```python
from build123d import *

# Parameters (mm, degrees)
SKETCH005_W     = 13
SKETCH005_H     = 11.2
SKETCH005_W_2   = 11.8
SKETCH005_H_2   = 10
PAD003_DEPTH    = 9.8
FILLET005_R     = 0.3
FILLET006_R     = 0.4
SKETCH006_W     = 1.85
SKETCH006_H     = 0.95
POCKET002_DEPTH = 0.6
FILLET007_R     = 0.13
SKETCH007_R     = 0.3
PAD004_DEPTH    = 1.3


with BuildPart() as part:
    # Sketch005 → Pad003 (new body)
    with BuildSketch(Plane.XY):
        with Locations((0, -1.6)):
            Rectangle(SKETCH005_W, SKETCH005_H)
        with Locations((0, -1.6)):
            Rectangle(SKETCH005_W_2, SKETCH005_H_2, mode=Mode.SUBTRACT)
    extrude(amount=PAD003_DEPTH)

    # Fillet005
    fillet005_edges = [part.edges().sort_by_distance(p)[0] for p in [
        (-6.5, 4, 4.9),
        (-6.5, -7.2, 4.9),
        (6.5, -7.2, 4.9),
        (6.5, 4, 4.9),
    ]]
    fillet(fillet005_edges, radius=FILLET005_R)

    # Fillet006
    fillet006_edges = [part.edges().sort_by_distance(p)[0] for p in [
        (-5.9, -6.6, 4.9),
        (-5.9, 3.4, 4.9),
        (5.9, -6.6, 4.9),
        (5.9, 3.4, 4.9),
    ]]
    fillet(fillet006_edges, radius=FILLET006_R)

    # Sketch006 (on Face10 of Fillet006) → Pocket002 (cut)
    with BuildSketch(Plane(origin=(0, 4, 0), x_dir=(-1, 0, 0), z_dir=(0, 1, 0))):
        with Locations((-3, 7.95)):
            Rectangle(SKETCH006_W, SKETCH006_H)
    pocket002 = extrude(amount=-POCKET002_DEPTH, mode=Mode.SUBTRACT)

    # Mirrored001: Pocket002 across Sketch006 V_Axis
    add(pocket002.mirror(Plane(origin=(0, 4, 0), x_dir=(0, 1, 0), z_dir=(-1, 0, 0))), mode=Mode.SUBTRACT)

    # Fillet007
    fillet007_edges = [part.edges().sort_by_distance(p)[0] for p in [
        (2.075, 3.7, 8.425),
        (2.075, 3.7, 7.475),
        (-3.925, 3.7, 7.475),
        (-3.925, 3.7, 8.425),
        (-2.075, 3.7, 8.425),
        (-2.075, 3.7, 7.475),
        (3.925, 3.7, 7.475),
        (3.925, 3.7, 8.425),
    ]]
    fillet(fillet007_edges, radius=FILLET007_R)

    # Sketch007 (on Face10 of Fillet007) → Pad004 (join)
    with BuildSketch(Plane(origin=(0, 0, 0), x_dir=(1, 0, 0), z_dir=(0, 0, -1))):
        with Locations((-6.1, 6.8)):
            Circle(SKETCH007_R)
        with Locations((6.1, 6.8)):
            Circle(SKETCH007_R)
        with Locations((-6.1, -3.6)):
            Circle(SKETCH007_R)
        with Locations((6.1, -3.6)):
            Circle(SKETCH007_R)
    extrude(amount=PAD004_DEPTH)


solid = part.part
```
Source: CAD feature listing. Evaluate the final solid. Frame: model axes, mm. A direction names the side the tool comes from. Round coordinates to 2 decimals unless told otherwise and drop trailing zeros. Write each loop counter-clockwise with the first axis right and the second up, starting at its lowest first coordinate (ties: lowest second). Pieces come first, ordered by that corner, then holes. Notation, with made-up numbers: M -30.75,33 L -6.75,33 A8 ccw -6.75,42 Z; hole C -5,78 d2. An arc over 180 degrees is marked long. Answer as a JSON object with one key per item and string values. Group by question number.
(1) Reachability of faces 4 (the flat face through (-5.9, -2, 5)), 5 (the flat face through (0, 3.8, 0)), 6 (the flat face through (0, -7.2, 5)) from +Z, -Z, +X, -X, +Y, -Y: full face, straight path, thin tool, end or side. Return the list, or none.
(2) Section query C-C on z = 3.5. Output: boundary loops of the cut face in (x, y).
(3) Mould query, pull axis X, two halves, no side actions, for faces 1 (the flat face through (-6.5, -2, 5)), 2 (the flat face through (0, 3.4, 5)), 3 (the flat face through (0, 4, 5)). Classes: +X half, -X half, draft (parallel to the pull), parting line (faces both ways), or undercut.
(4) Section query A-A on y = 2.25. Output: boundary loops of the cut face in (x, z).
(5) Ray query, line 1 (X direction, y = -2.5, z = 5.25); line 2 (Y direction, x = 2.75, z = 0.25); line 3 (Z direction, x = -6, y = 2.75). Return the intervals inside material, ascending. Write a range as [from, to].
(6) Section query B-B on x = 0. Output: boundary loops of the cut face in (y, z), then the cut area to 3 significant figures.
(7) First-contact query: pin 1 (2 mm diameter, centred on x = 5, y = -4.5, fed in from +Z). Flat tip, straight axial feed; report the tip coordinate or a pass-through.
Computed values:
{
 "1": {"face 4": "+Z, -Z", "face 5": "-Z", "face 6": "+Z, -Z, +X, -X, -Y"},
 "2": {"outline": "M -6.5,-6.9 A0.3 ccw -6.2,-7.2 L 6.2,-7.2 A0.3 ccw 6.5,-6.9 L 6.5,3.7 A0.3 ccw 6.2,4 L -6.2,4 A0.3 ccw -6.5,3.7 Z; hole M -5.9,-6.2 A0.4 ccw -5.5,-6.6 L 5.5,-6.6 A0.4 ccw 5.9,-6.2 L 5.9,3 A0.4 ccw 5.5,3.4 L -5.5,3.4 A0.4 ccw -5.9,3 Z"},
 "3": {"face 1": "-X half", "face 2": "undercut", "face 3": "draft"},
 "4": {"outline": "M -6.5,0 L -5.9,0 L -5.9,9.8 L -6.5,9.8 Z; M 5.9,0 L 6.5,0 L 6.5,9.8 L 5.9,9.8 Z"},
 "5": {"line 1": "[-6.5, -5.9], [5.9, 6.5]", "line 2": "[-7.2, -6.6], [3.4, 4]", "line 3": "[0, 9.8]"},
 "6": {"outline": "M -7.2,0 L -6.6,0 L -6.6,9.8 L -7.2,9.8 Z; M 3.4,0 L 4,0 L 4,9.8 L 3.4,9.8 Z", "area": "11.8 mm^2"},
 "7": {"pin 1": "z = 9.8"}
}
